Geometry: see drawing. Coordinates: mm, zero at the bounding-box minimum. A direction names the side the tool comes from. Coordinates: 2 decimals unless noted, no trailing zeros. Order: outer loops, then holes, each group sorted by start corner. A loop starts at its lowest first (then second) coordinate and runs counter-clockwise, first axis right, second up. Notation, with made-up numbers: (-5, 15) -> (31, 15) arc R14 ccw to (31, 34) -> close; hole circle Ø7 at (24.25, 34). An arc over 180 degrees is marked (long way). Use CSV: the item, a comma, the result in double quotes. Start each with the question number.
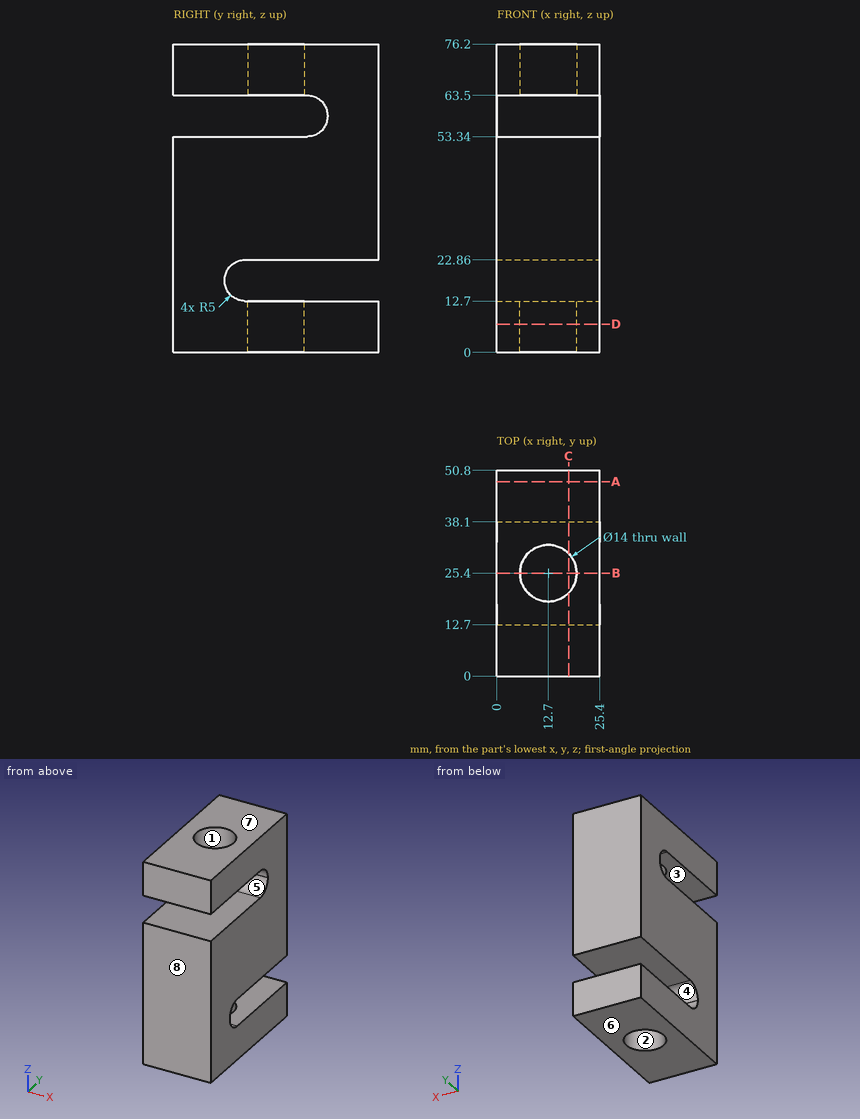
(1) First-contact query: pin 1 (12.5 mm diameter, centred on x = 12.7, y = 25.4, fed in from +Z). Flat tip, straight axial feed; report the tip coordinate or a pass-through.
(2) Line query: line 1 (Z direction, x = 4.5, y = 29); line 2 (Y direction, x = 12.7, z = 5.75); line 3 (Z direction, x = 9.75, y = 8). Output: solid intervals per line, ascending. Write a range as from..to.
(3) Mould query, pull axis Z, two halves, no side actions, for the marked faces 5, 6, 7 and 8. Classes: pulls with the +Z half, pulls with the -Z half, needs draft (parallel to the pull), parting line crosses it, or undercut.
(4) Access query for the marked faces 1, 2, 3 and 4. Directions: +Z, -Z, +X, -X, +Y, -Y. A direction counts if a zero-diameter tool reaches every point of the face in a straight line with its end or side. Return the directions, or none.
(5) Section D-D (z = 7). Return loops of the section in (x, y).
(6) Section B-B (y = 25.4). Return loops of the section in (x, z), then the cut area to 3 significant figures.
(7) Section C-C (x = 17.75). Return loops of the section in (y, z).
(8) Section A-A (y = 48). Return loops of the section in (x, z), then the cut area to 3 significant figures.
Check sheet entries:
1,pin 1,"stops at z = 53.34"
2,line 1,"z = 0..12.7, 22.86..53.34, 63.5..76.2"
2,line 2,"y = 0..18.4, 32.4..50.8"
2,line 3,"z = 0..53.34, 63.5..76.2"
3,face 5,"undercut"
3,face 6,"pulls with the -Z half"
3,face 7,"pulls with the +Z half"
3,face 8,"needs draft"
4,face 1,"+Z"
4,face 2,"-Z"
4,face 3,"+X, -X, -Y"
4,face 4,"+X, -X, +Y"
5,outline,"(0, 0) -> (25.4, 0) -> (25.4, 50.8) -> (0, 50.8) -> close; hole circle Ø14 at (12.7, 25.4)"
6,outline,"(0, 0) -> (5.7, 0) -> (5.7, 12.7) -> (0, 12.7) -> close; (0, 22.86) -> (25.4, 22.86) -> (25.4, 53.34) -> (0, 53.34) -> close; (0, 63.5) -> (5.7, 63.5) -> (5.7, 76.2) -> (0, 76.2) -> close; (19.7, 0) -> (25.4, 0) -> (25.4, 12.7) -> (19.7, 12.7) -> close; (19.7, 63.5) -> (25.4, 63.5) -> (25.4, 76.2) -> (19.7, 76.2) -> close"
6,area,"1,060 mm^2"
7,outline,"(0, 0) -> (20.55, 0) -> (20.55, 12.7) -> (17.7, 12.7) arc R5 cw to (12.7, 17.7) -> (12.7, 17.86) arc R5 cw to (17.7, 22.86) -> (50.8, 22.86) -> (50.8, 76.2) -> (30.25, 76.2) -> (30.25, 63.5) -> (33.1, 63.5) arc R5 cw to (38.1, 58.5) -> (38.1, 58.34) arc R5 cw to (33.1, 53.34) -> (0, 53.34) -> close; (0, 63.5) -> (20.55, 63.5) -> (20.55, 76.2) -> (0, 76.2) -> close; (30.25, 0) -> (50.8, 0) -> (50.8, 12.7) -> (30.25, 12.7) -> close"
8,outline,"(0, 0) -> (25.4, 0) -> (25.4, 12.7) -> (0, 12.7) -> close; (0, 22.86) -> (25.4, 22.86) -> (25.4, 76.2) -> (0, 76.2) -> close"
8,area,"1,680 mm^2"
